Here's how the part is built. I have some questions about the finished solid (model axes, mm). A direction names the side the tool comes from. Coordinates: 2 decimals unless noted, no trailing zeros. Loops run counter-clockwise (first coordinate to the right, second up) from the corner with the lowest first, then second, coordinate; pieces in that order, holes last. Notation, with made-up numbers: (20, -6.5) -> (45, -6.5) arc R13 ccw to (45, 10.5) -> close; hole circle Ø3 at (-20, 27). An arc over 180 degrees is marked (long way). Answer as a JSON object with one key per item and string values. Group by question number.
1) Which directions (+Z, -Z, +X, -X, +Y, -Y) give clear straight access to the entire face, cutting with the end or side of a thin tool? Please do faces 1 (the flat face through (7.366, 82, 70)), 2 (the flat face through (5.75, 80, 70)), 3 (the cylindrical face through (-46.8, -47.6, 7.6)), 4 (the flat face through (0, -24.8, 27)), 5 (the flat face through (-7.366, 82, 70)).
2) I want a section at B-B (x = -50). Write out the boundary of the cut face in (y, z).
3) I need wall thicknesses on probe 1 along Y at (x, z) = (50, 8.5); probe 2 along X at (y, z) = (-50, 10.5); probe 3 along Y at (x, z) = (-39.5, 71.5). Which ranges of each line are inside material? Lowest first, please. Write a range as [from, to].
4) I want a section at A-A (z = 24). Write out the boundary of the cut face in (x, y), then the cut area to 4 significant figures.
5) I want a section at C-C (y = 50). Write out the boundary of the cut face in (x, z), then the cut area to 3 significant figures.
6) I want a section at D-D (z = 12). Write out the boundary of the cut face in (x, y).
7) I'm going to push flat-ended pins straight in: pin 1 (3 mm diameter, centred on y = 80, z = 68, fed in from -X); pin 2 (2.5 mm diameter, centred on y = 83.5, z = 75.5, fed in from +X); pin 3 (8 mm diameter, centred on x = -34.5, y = -5, fed in from +Z). Where does each tip first touch, or does it pass through?
8) If we mould it in two halves opening along Y, with no side actions, what happens to faces 6 (the flat face through (-85, -1, 49)), 7 (the flat face through (-1, -80, 49)), 8 (the flat face through (-16.4, 21.2, 40))? For each: +Y half, -Y half, draft (parallel to the pull), parting line (faces both ways), or undercut.
```python
from build123d import *

# Parameters (mm, degrees)
F0_W      = 170
F0_H      = 160
F1_DEPTH  = 100
F2_W      = 160
F2_H      = 150
F3_DEPTH  = 85
F4_W      = 14.732
F4_H      = 50
F5_DEPTH  = 5
F6_W      = 11.5
F6_H      = 47.5
F7_DEPTH  = 10
F8_R      = 2.5
F9_W      = 55
F9_H      = 55
F10_DEPTH = 25
F11_R     = 25
F12_DEPTH = 5
F14_D     = 8


with BuildPart() as f1:
    # F0 (on Top) → F1 (new body)
    with BuildSketch(Plane.XY):
        Rectangle(F0_W, F0_H)
    extrude(amount=F1_DEPTH)

    # F2 (on face) → F3 (cut)
    with BuildSketch(Plane.XY.offset(100)):
        Rectangle(F2_W, F2_H)
    extrude(amount=-F3_DEPTH, mode=Mode.SUBTRACT)

    # F4 (on face) → F5 (join)
    with BuildSketch(Plane(origin=(0, 80, 0), x_dir=(-1, 0, 0), z_dir=(0, 1, 0))):
        with Locations((0, 70)):
            Rectangle(F4_W, F4_H)
    extrude(amount=F5_DEPTH)

    # F6 (on face) → F7 (cut, through all)
    with BuildSketch(Plane(origin=(0, 85, 0), x_dir=(-1, 0, 0), z_dir=(0, 1, 0))):
        with Locations((0, 70)):
            Rectangle(F6_W, F6_H)
    extrude(amount=-F7_DEPTH, mode=Mode.SUBTRACT)

    # F8
    f8_edges = [f1.edges().sort_by_distance(p)[0] for p in [
        (85, -80, 50),
        (-85, -80, 50),
        (85, 80, 50),
        (-85, 80, 50),
        (80, 75, 57.5),
        (-80, 75, 57.5),
        (-80, -75, 57.5),
        (80, -75, 57.5),
    ]]
    fillet(f8_edges, radius=F8_R)

    # F9 (on face) → F10 (join)
    with BuildSketch(Plane.XY.offset(15)):
        with Locations((0, 2.7)):
            Rectangle(F9_W, F9_H)
    extrude(amount=F10_DEPTH)

    # F11 (on face) → F12 (cut)
    with BuildSketch(Plane.XY.offset(40)):
        with Locations((0, 2)):
            Circle(F11_R)
    extrude(amount=-F12_DEPTH, mode=Mode.SUBTRACT)

    # F14 (through all)
    with Locations(Plane(origin=(0, 0, 0), x_dir=(1, 0, 0), z_dir=(0, 0, -1))):
        with Locations((-50, 50), (50, 50), (50, -50), (-50, -50)):
            Hole(F14_D / 2)


solid = f1.part
```
Determined:
{
 "1": {"face 1": "+Z, -Z, +X, +Y", "face 2": "+Y", "face 3": "+Z, -Z", "face 4": "+Z", "face 5": "+Z, -Z, -X, +Y"},
 "2": {"outline": "(-80, 0) -> (-54, 0) -> (-54, 15) -> (-75, 15) -> (-75, 100) -> (-80, 100) -> close; (-46, 0) -> (46, 0) -> (46, 15) -> (-46, 15) -> close; (54, 0) -> (80, 0) -> (80, 100) -> (75, 100) -> (75, 15) -> (54, 15) -> close"},
 "3": {"probe 1": "[-80, -54], [-46, 46], [54, 80]", "probe 2": "[-85, -54], [-46, 46], [54, 85]", "probe 3": "[-80, -75], [75, 80]"},
 "4": {"outline": "(-85, -77.5) arc R2.5 ccw to (-82.5, -80) -> (82.5, -80) arc R2.5 ccw to (85, -77.5) -> (85, 77.5) arc R2.5 ccw to (82.5, 80) -> (-82.5, 80) arc R2.5 ccw to (-85, 77.5) -> close; (-27.5, -24.8) -> (27.5, -24.8) -> (27.5, 30.2) -> (-27.5, 30.2) -> close; hole (-80, -72.5) arc R2.5 ccw to (-77.5, -75) -> (77.5, -75) arc R2.5 ccw to (80, -72.5) -> (80, 72.5) arc R2.5 ccw to (77.5, 75) -> (-77.5, 75) arc R2.5 ccw to (-80, 72.5) -> close", "area": "6,225 mm^2"},
 "5": {"outline": "(-85, 0) -> (-54, 0) -> (-54, 15) -> (-80, 15) -> (-80, 100) -> (-85, 100) -> close; (-46, 0) -> (46, 0) -> (46, 15) -> (-46, 15) -> close; (54, 0) -> (85, 0) -> (85, 100) -> (80, 100) -> (80, 15) -> (54, 15) -> close", "area": "3,160 mm^2"},
 "6": {"outline": "(-85, -77.5) arc R2.5 ccw to (-82.5, -80) -> (82.5, -80) arc R2.5 ccw to (85, -77.5) -> (85, 77.5) arc R2.5 ccw to (82.5, 80) -> (-82.5, 80) arc R2.5 ccw to (-85, 77.5) -> close; hole circle Ø8 at (-50, -50); hole circle Ø8 at (-50, 50); hole circle Ø8 at (50, -50); hole circle Ø8 at (50, 50)"},
 "7": {"pin 1": "x = -84.79", "pin 2": "x = 7.37", "pin 3": "z = 15"},
 "8": {"face 6": "draft", "face 7": "-Y half", "face 8": "undercut"}
}
